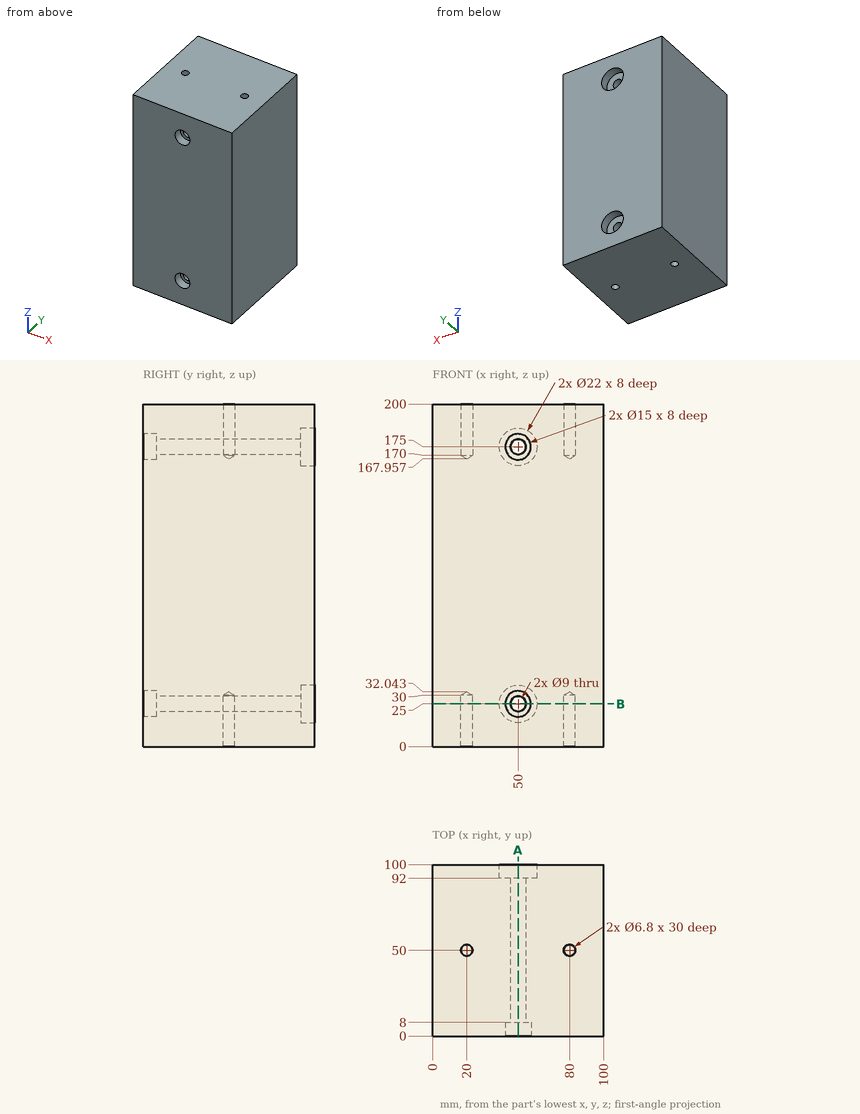
Print and shaded views of the part. All mm, measured from the part's lowest x, y and z. Round coordinates to 2 decimals unless told otherwise and drop trailing zeros. Loops run counter-clockwise (first coordinate to the right, second up) from the corner with the lowest first, then second, coordinate; pieces in that order, holes last. Notation, with made-up numbers: M 7,-9 L 27,-9 A31 cw 27,30 Z; hole C -11,78.25 d3. An arc over 180 degrees is marked long. One line per question, with ' | ' between items.
1) Band-saw the part on A-A (x = 50). Give the cut face in (y, z).
Solved:
outline: M 0,0 L 100,0 L 100,14 L 92,14 L 92,20.5 L 8,20.5 L 8,17.5 L 0,17.5 Z; M 0,32.5 L 8,32.5 L 8,29.5 L 92,29.5 L 92,36 L 100,36 L 100,164 L 92,164 L 92,170.5 L 8,170.5 L 8,167.5 L 0,167.5 Z; M 0,182.5 L 8,182.5 L 8,179.5 L 92,179.5 L 92,186 L 100,186 L 100,200 L 0,200 Z
2) Band-saw the part on B-B (z = 25). Give the cut face in (x, y).
Solved:
outline: M 0,0 L 42.5,0 L 42.5,8 L 45.5,8 L 45.5,92 L 39,92 L 39,100 L 0,100 Z; M 54.5,8 L 57.5,8 L 57.5,0 L 100,0 L 100,100 L 61,100 L 61,92 L 54.5,92 Z; hole C 20,50 d6.8; hole C 80,50 d6.8
3) Flat gauge pins, fed straight in: pin 1 (17 mm diameter, centred on x = 50, z = 25, fed in from +Y); pin 2 (5.5 mm diameter, centred on x = 20, y = 50, fed in from -Z); pin 3 (7.5 mm diameter, centred on x = 48.5, z = 25, fed in from -Y). Where does each tip first touch, or does it go through?
Solved:
pin 1: stops at y = 92 | pin 2: stops at z = 30.39 | pin 3: stops at y = 8
4) Drill centre lines: line 1 along Z through (x, y) = (50, 96); line 2 along X through (y, z) = (78.5, 178); line 3 along X through (y, z) = (2, 175). Where is each one in solid material? Low to high.
Solved:
line 1: z = 0 to 14, 36 to 164, 186 to 200 | line 2: x = 0 to 46.65, 53.35 to 100 | line 3: x = 0 to 42.5, 57.5 to 100
